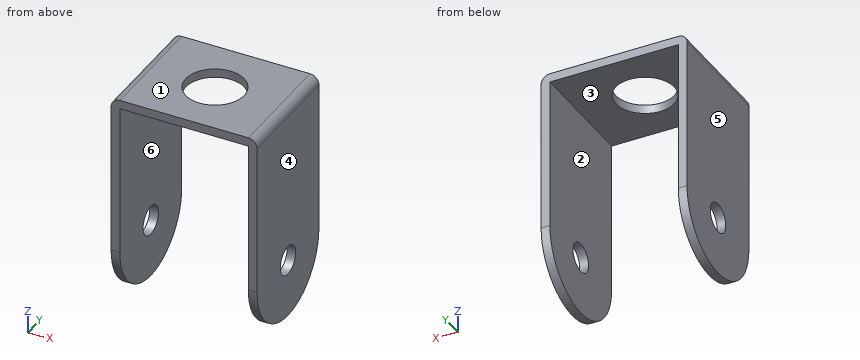
Autodesk Inventor part; units mm, degrees
ref_plane "YZ Plane" through (0, 0, 0) normal (1, 0, 0) x (0, 1, 0)
ref_plane "XZ Plane" through (0, 0, 0) normal (0, 1, 0) x (-1, 0, 0)
ref_plane "XY Plane" through (0, 0, 0) normal (0, 0, 1) x (1, 0, 0)
sketch "Sketch1" plane through (0, 0, 0) normal (0, 1, 0) x (-1, 0, 0)
  line L0 (50, 0) -> (50, 75)
  line L1 (50, 75) -> (0, 75)
  line L2 (0, 75) -> (0, 0)
  line L3 (3, 0) -> (3, 72)
  line L4 (3, 72) -> (47, 72)
  line L5 (47, 72) -> (47, 0)
  line L6 (0, 0) -> (3, 0)
  line L7 (47, 0) -> (50, 0)
  dimension "d0" = 50
  dimension "d1" = 75
  dimension "d2" = 3
extrude "Extrusion1" add sketch "Sketch1" along normal mid plane 40
fillet "Fillet1" radius 20 4 edges at (-48.5, 20, 0) (-48.5, -20, 0) (-1.5, 20, 0) (-1.5, -20, 0)
fillet "Fillet2" radius 3 2 edges at (-50, 0, 75) (0, 0, 75)
sketch "Sketch2" plane through (-50, 0, 20) normal (-1, 0, 0) x (0, 0, 1)
  circle A0 centre (0, 0) radius 5
  point P0 (-20, 0)
  dimension "d7" = 10
extrude "Extrusion2" cut sketch "Sketch2" against normal through all
sketch "Sketch3" plane through (-47, 20, 75) normal (0, 0, 1) x (1, 0, 0)
  circle A0 centre (22, -20) radius 10
  point P0 (47, -20)
  dimension "d10" = 20
extrude "Extrusion3" cut sketch "Sketch3" against normal blind 10
Read the model definition and answer for the solid it produces. Units are mm, in the model's axes. Face numbers are marked on the shaded views. A direction names the side the tool comes from. Coordinates: 2 decimals unless noted, no trailing zeros. Order: outer loops, then holes, each group sorted by start corner. A loop starts at its lowest first (then second) coordinate and runs counter-clockwise, first axis right, second up. Notation, with made-up numbers: M 8,-17 L 65,-17 A5 cw 65,-12 Z; hole C 61,7 d1. An arc over 180 degrees is marked long. Put each result on its own line as item: value. Start each with the question number.
Item 1: Section B-B, the plane z = 70 is taken. Determine the outline of the cut face in (x, y).
Item 2: For the marked faces 1 and 2, determine the directions among +Z, -Z, +X, -X, +Y, -Y from which every point of the face is accessible in a straight line to the end or side of a thin tool.
Item 3: The mould has two halves that part along X. Classify the marked faces 3, 4, 5 and 6: +X half, -X half, draft (parallel to the pull), parting line (faces both ways), or undercut.
Item 4: Consider probe 1 along X at (y, z) = (-16, 33); probe 2 along Y at (x, z) = (-48.6, 20); probe 3 along Y at (x, z) = (-25, 73.6). Determine where each line is inside the solid, lowest interval first. Write a range as [from, to].
Item 5: Section A-A, the plane x = -17 is taken. Determine the outline of the cut face in (y, z).
Item 6: Given pin 1 Ø9 at (y, z) = (0, 20) entering from -X, flat-ended and moving along its own axis, determine where the tip first touches the part or whether it passes through.
Item 7: Section C-C, the plane z = 16 is taken. Determine the outline of the cut face in (x, y).
Item 8: Section D-D, the plane x = -6.5 is taken. Determine the outline of the cut face in (y, z), plus the area to 3 significant figures.
Computed:
1. outline: M -50,-20 L -47,-20 L -47,20 L -50,20 Z; M -3,-20 L 0,-20 L 0,20 L -3,20 Z
2. face 1: +Z, +X, -X, +Y, -Y
2. face 2: -Z, +Y, -Y
3. face 3: undercut
3. face 4: +X half
3. face 5: -X half
3. face 6: undercut
4. probe 1: x = [-50, -47], [-3, 0]
4. probe 2: y = [-20, -5], [5, 20]
4. probe 3: y = [-20, -10], [10, 20]
5. outline: M -20,72 L -6,72 L -6,75 L -20,75 Z; M 6,72 L 20,72 L 20,75 L 6,75 Z
6. pin 1: passes through
7. outline: M -50,-19.6 L -47,-19.6 L -47,-3 L -50,-3 Z; M -50,3 L -47,3 L -47,19.6 L -50,19.6 Z; M -3,-19.6 L 0,-19.6 L 0,-3 L -3,-3 Z; M -3,3 L 0,3 L 0,19.6 L -3,19.6 Z
8. outline: M -20,72 L 20,72 L 20,75 L -20,75 Z
8. area: 120 mm2
